Could you check a few things on this model? Use its own coordinates, in mm. A direction names the side the tool comes from. Coordinates: 2 decimals unless noted, no trailing zeros. Write each loop counter-clockwise with the first axis right and the second up, starting at its lowest first coordinate (ties: lowest second). Pieces come first, ordered by that corner, then holes. Notation, with made-up numbers: (12, 85) - (30, 85) arc R29 cw to (30, 109) - close; hole circle Ø5 at (61, 25.5). An arc over 180 degrees is marked (long way). Answer as a JSON object with one key per item and string values. Group by question number.
1) On a 3-axis mill with a long thin cutter (end or side, diameter ignored), from which of +Z, -Z, +X, -X, +Y, -Y can I reach the whole of each face in a straight line? I mean faces 1 (the flat face through (-266.66, 265, 862)), 2 (the flat face through (-464, 341, 780)), 3 (the flat face through (-464, 400, 831)). Say none if no direction works.
2) If we section it at B-B (x = -1558): Write out the boundary of the cut face in (y, z), plus the area to 3 significant figures.
3) If we section it at D-D (y = 501): Write out the boundary of the cut face in (x, z), plus the area to 3 significant figures.
4) Will these pins go through, and if not, where does the flat tip stop? pin 1 Ø1.5 at (x, y) = (-906.5, 324) entering from +Z; pin 2 Ø22 at (y, z) = (15, 437) entering from +X; pin 3 Ø3 at (y, z) = (410, 388.5) entering from +X.
5) Please list where these lines run through material, in increasing order: line 1 along Y through (x, z) = (-1018, 968); line 2 along X through (y, z) = (231, 528); line 3 along Z through (x, y) = (-1732.5, 437).
6) If we section it at C-C (z = 635): Write out the boundary of the cut face in (x, y), plus the area to 3 significant figures.
7) If we section it at A-A (y = 171): Write out the boundary of the cut face in (x, z), plus the area to 3 significant figures.
8) We'd pull the mould along X, two halves only. Please class faces 4 (the flat face through (-20, 286, 974)), 5 (the flat face through (-936, 20, 866)), 6 (the flat face through (-463.9, 181.4, 849.3)), 7 (the flat face through (0, 296, 971)): released by +X, released by -X, zero draft, split by the parting line, or undercut.
```python
from build123d import *

# Parameters (mm, degrees)
SKETCH002_W      = 1880
SKETCH002_H      = 880
EXTRUDE002_DEPTH = 580
SKETCH001_W      = 1850
SKETCH001_H      = 850
EXTRUDE001_DEPTH = 20
SKETCH003_W      = 400
SKETCH003_H      = 300
EXTRUDE003_DEPTH = 20
SKETCH004_W      = 1900
SKETCH004_H      = 150
EXTRUDE004_DEPTH = 20
SKETCH005_W      = 20
SKETCH005_H      = 150
EXTRUDE005_DEPTH = 600
SKETCH_W         = 1900
SKETCH_H         = 900
EXTRUDE_DEPTH    = 600
EXTRUDE006_DEPTH = 400
EXTRUDE007_DEPTH = 440


with BuildPart() as base:
    # Sketch002 → Extrude002 (new body)
    with BuildSketch(Plane.XZ):
        with Locations((940, 440)):
            Rectangle(SKETCH002_W, SKETCH002_H)
    extrude(amount=-EXTRUDE002_DEPTH)


with BuildPart() as base_1:
    # Extrude002 placement: moved
    add(base.part.moved(Location((0, 20, 0))))


with BuildPart() as obj1:
    # Sketch001 → Extrude001 (new body)
    with BuildSketch(Plane.XZ):
        with Locations((925, 425)):
            Rectangle(SKETCH001_W, SKETCH001_H)
    extrude(amount=-EXTRUDE001_DEPTH)


with BuildPart() as obj2:
    # Sketch003 → Extrude003 (new body)
    with BuildSketch(Plane.XY):
        with Locations((200, 150)):
            Rectangle(SKETCH003_W, SKETCH003_H)
    extrude(amount=EXTRUDE003_DEPTH)


with BuildPart() as obj2_1:
    # Extrude003 placement: moved
    add(obj2.part.moved(Location((266.66, 80, 880))))

    # Fusion: union Base , obj1
    add(base_1.part)
    add(obj1.part)


with BuildPart() as obj3:
    # Sketch004 → Extrude004 (new body)
    with BuildSketch(Plane.XZ):
        with Locations((950, 75)):
            Rectangle(SKETCH004_W, SKETCH004_H)
    extrude(amount=EXTRUDE004_DEPTH)


with BuildPart() as obj3_1:
    # Extrude004 placement: moved
    add(obj3.part.moved(Location((0, 600, 900))))


with BuildPart() as extrude005:
    # Sketch005 → Extrude005 (new body)
    with BuildSketch(Plane.XZ):
        with Locations((10, 75)):
            Rectangle(SKETCH005_W, SKETCH005_H)
    extrude(amount=-EXTRUDE005_DEPTH)


with BuildPart() as extrude005_1:
    # Extrude005 placement: moved
    add(extrude005.part.moved(Location((0, 0, 900))))


with BuildPart() as cut:
    # Sketch → Extrude (new body)
    with BuildSketch(Plane.XZ):
        with Locations((950, 450)):
            Rectangle(SKETCH_W, SKETCH_H)
    extrude(amount=-EXTRUDE_DEPTH)

    # Fusion001: union obj3 , Extrude005
    add(obj3_1.part)
    add(extrude005_1.part)

    # Cut: cut obj2
    add(obj2_1.part, mode=Mode.SUBTRACT)


with BuildPart() as extrude006:
    # Sketch006 → Extrude006 (new body)
    with BuildSketch(Plane.YZ):
        Polygon((0, 0), (300, 0), (300, -100), (200, -100), align=None)
    extrude(amount=EXTRUDE006_DEPTH)


with BuildPart() as obj4:
    # Sketch007 → Extrude007 (new body)
    with BuildSketch(Plane.YZ):
        Polygon((-40, 0), (320, 0), (320, -120), (200, -120), align=None)
    extrude(amount=EXTRUDE007_DEPTH)


with BuildPart() as obj4_1:
    # Extrude007 placement: moved
    add(obj4.part.moved(Location((-20, 0, 0))))

    # Cut001: cut Extrude006
    add(extrude006.part, mode=Mode.SUBTRACT)


with BuildPart() as obj4_2:
    # Cut001 placement: moved
    add(obj4_1.part.moved(Location((266.66, 80, 900))))

    # Fusion015: union Cut
    add(cut.part)


with BuildPart() as mirror:
    # Mirror: instance of obj4
    add(obj4_2.part.mirror(Plane(origin=(0, 0, 0), x_dir=(0, -1, 0), z_dir=(1, 0, 0))))


solid = mirror.part
```
Here are the results:
{
 "1": {"face 1": "+Z", "face 2": "-Z, +X, +Y, -Y", "face 3": "-Z, +X, +Y"},
 "2": {"outline": "(0, 850) - (20, 850) - (20, 880) - (600, 880) - (600, 1050) - (580, 1050) - (580, 900) - (0, 900) - close", "area": "15,600 mm²"},
 "3": {"outline": "(-1900, 0) - (-1880, 0) - (-1880, 880) - (0, 880) - (0, 1050) - (-20, 1050) - (-20, 900) - (-1900, 900) - close", "area": "58,600 mm²"},
 "4": {"pin 1": "stops at z = 900", "pin 2": "stops at x = -1850", "pin 3": "stops at x = -1880"},
 "5": {"line 1": "y = 580 to 600", "line 2": "x = -1900 to -1880", "line 3": "z = 880 to 900"},
 "6": {"outline": "(-1900, 0) - (-1850, 0) - (-1850, 20) - (-1880, 20) - (-1880, 600) - (-1900, 600) - close", "area": "12,600 mm²"},
 "7": {"outline": "(-1900, 0) - (-1880, 0) - (-1880, 880) - (-686.66, 880) - (-686.66, 834.5) - (-246.66, 834.5) - (-246.66, 880) - (0, 880) - (0, 1050) - (-20, 1050) - (-20, 900) - (-266.66, 900) - (-266.66, 854.5) - (-666.66, 854.5) - (-666.66, 900) - (-1900, 900) - close", "area": "60,400 mm²"},
 "8": {"face 4": "released by -X", "face 5": "zero draft", "face 6": "undercut", "face 7": "released by +X"}
}
